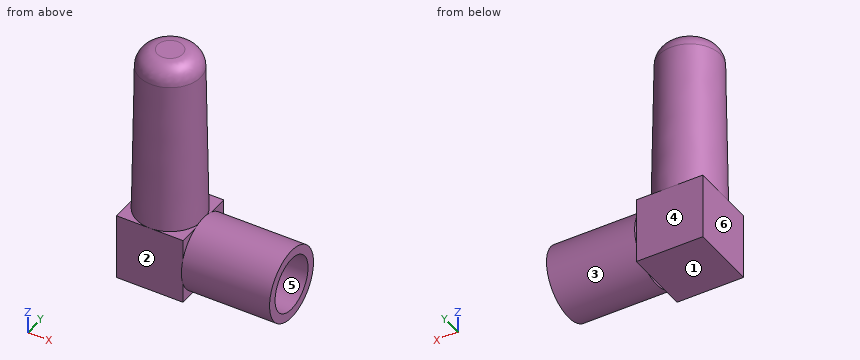
Autodesk Inventor part; units mm, degrees
ref_plane "YZ Plane" through (0, 0, 0) normal (1, 0, 0) x (0, 1, 0)
ref_plane "XZ Plane" through (0, 0, 0) normal (0, 1, 0) x (-1, 0, 0)
ref_plane "XY Plane" through (0, 0, 0) normal (0, 0, 1) x (1, 0, 0)
sketch "Skizze1" plane through (0, 0, 0) normal (0, 0, 1) x (1, 0, 0)
  line L0 (-3.7, 3.7) -> (3.7, 3.7)
  line L1 (3.7, 3.7) -> (3.7, -3.7)
  line L2 (3.7, -3.7) -> (-3.7, -3.7)
  line L3 (-3.7, -3.7) -> (-3.7, 3.7)
  line L4 (0, 5.18) -> (0, -5.18)
  line L5 (-5.18, 0) -> (5.18, 0)
  point P0 (0, 0)
  dimension "d0" = 7.4
  dimension "d1" = 7.4
extrude "Extrusion1" add sketch "Skizze1" against normal blind 7.4
sketch "Skizze2" plane through (0, 0, 0) normal (0, 0, 1) x (1, 0, 0)
  circle A0 centre (0, 0) radius 3.7
  dimension "d4" = 7.4
extrude "Extrusion2" add sketch "Skizze2" along normal blind 19 draft -1
fillet "Rundung1" radius 2 1 edges at (-3.3684, 0, 19)
sketch "Skizze3" plane through (3.7, -3.7, -7.4) normal (1, 0, 0) x (0, 0, -1)
  line L0 (-7.4, 7.4) -> (-7.4, 3.7)
  line L1 (-7.4, 3.7) -> (-7.4, 0)
  line L2 (-7.4, 0) -> (0, 0)
  line L3 (0, 7.4) -> (0, 0)
  line L4 (-7.4, 7.4) -> (0, 7.4)
  line L5 (-7.4, 3.7) -> (0, 3.7) construction
  line L6 (0, 7.4) -> (0, 0) construction
  line L7 (-7.4, 0) -> (0, 0) construction
  line L8 (-3.7, 0) -> (-3.7, 7.4) construction
  line L9 (-7.4, 7.4) -> (0, 7.4) construction
  circle A0 centre (-3.7, 3.7) radius 4
  circle A1 centre (-3.7, 3.7) radius 3
  dimension "d8" = 8
  dimension "d9" = 6
extrude "Extrusion3" add sketch "Skizze3" along normal blind 9.8 contours A0 L4 L3 L2 L1 L0 | L0 L1 A0 | A0 L4 | L2 A0 | A0 L3
properties part number "Antenne-Klein" material "Aluminium 6061"
Geometry: final body of the model. Coordinates: model frame, mm. Face numbers are marked on the shaded views. A direction names the side the tool comes from. Round coordinates to 2 decimals unless told otherwise and drop trailing zeros. Loops run counter-clockwise (first coordinate to the right, second up) from the corner with the lowest first, then second, coordinate; pieces in that order, holes last. Notation, with made-up numbers: (55, 40.5) -> (88, 40.5) arc R18 cw to (88, 48.5) -> close; hole circle Ø8 at (26.5, 44.5). An arc over 180 degrees is marked (long way). One line per question, with ' | ' between items. Start each with the question number.
1. Mould query, pull axis Y, two halves, no side actions, for the marked faces 4, 5 and 6. Classes: pulls with the +Y half, pulls with the -Y half, needs draft (parallel to the pull), parting line crosses it, or undercut.
2. Contact query for flat-ended pins moving along their axis: pin 1 (4 mm diameter, centred on x = -2.5, y = -2.5, fed in from +Z); pin 2 (6 mm diameter, centred on x = -0.5, z = -2, fed in from +Y); pin 3 (6 mm diameter, centred on x = -1, z = -4, fed in from -Y); pin 4 (2.5 mm diameter, centred on y = -3, z = -0.5, fed in from +X). Output: stop coordinate, or through.
3. Section C-C on z = 9.25. Output: boundary loops of the cut face in (x, y), and give its area (3 significant figures).
4. Line query: line 1 along Y through (x, z) = (8.25, -3.7); line 2 along Y through (x, z) = (0, 16.75); line 3 along Z through (x, y) = (10, 0.25). Output: solid intervals per line, ascending. Write a range as [from, to].
5. Section A-A on z = -3.7. Output: boundary loops of the cut face in (x, y), and give its area (3 significant figures).
6. Section B-B on z = -1. Output: boundary loops of the cut face in (x, y).
7. Section D-D on z = 6.25. Output: boundary loops of the cut face in (x, y).
8. Set-up query: the marked faces 1, 2 and 3. Return all of +Z, -Z, +X, -X, +Y, -Y with unobstructed straight access to the full face (end or side cutting, diameter ignored); none if empty.
Returned:
1) face 4: pulls with the +Y half | face 5: undercut | face 6: needs draft
2) pin 1: stops at z = 19 | pin 2: stops at y = 3.7 | pin 3: stops at y = -3.7 | pin 4: stops at x = 13.5
3) outline: circle Ø7.08 at (0, 0) | area: 39.3 mm2
4) line 1: y = [-4, -3], [3, 4] | line 2: y = [-3.41, 3.41] | line 3: z = [-7.69, -6.69], [-0.71, 0.29]
5) outline: (-3.7, -3.7) -> (3.7, -3.7) -> (3.7, -4) -> (13.5, -4) -> (13.5, -3) -> (3.7, -3) -> (3.7, 3) -> (13.5, 3) -> (13.5, 4) -> (3.7, 4) -> (3.7, 3.7) -> (-3.7, 3.7) -> close | area: 74.4 mm2
6) outline: (-3.7, -3.7) -> (3.7, -3.7) -> (3.7, -2.95) -> (13.5, -2.95) -> (13.5, -1.31) -> (3.7, -1.31) -> (3.7, 1.31) -> (13.5, 1.31) -> (13.5, 2.95) -> (3.7, 2.95) -> (3.7, 3.7) -> (-3.7, 3.7) -> close
7) outline: circle Ø7.18 at (0, 0)
8) face 1: -Z, -X, +Y, -Y | face 2: +Z, -Z, -X, -Y | face 3: +X
